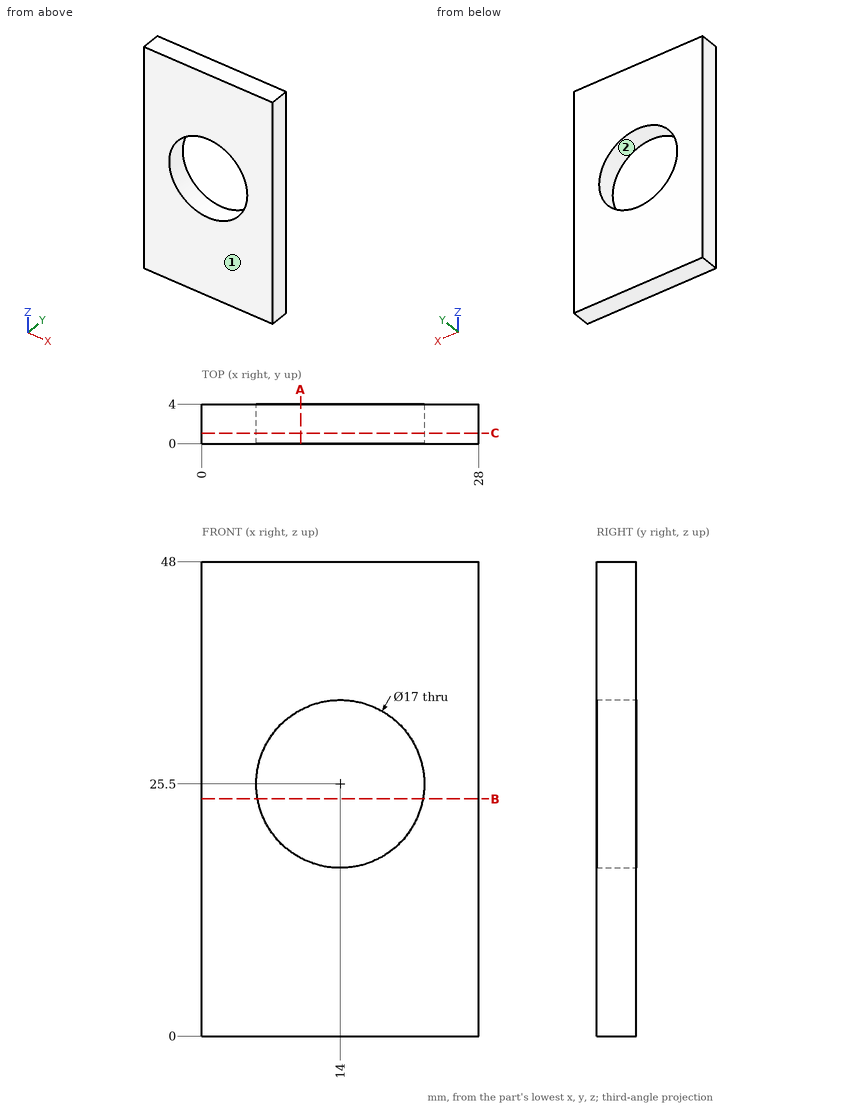
Design review of the part shown in the three views and the two pictorial views. Dimensions are in mm from the part's minimum x, y and z. Round coordinates to 2 decimals unless told otherwise and drop trailing zeros. Order: outer loops, then holes, each group sorted by start corner. A loop starts at its lowest first (then second) coordinate and runs counter-clockwise, first axis right, second up.
(1) Take a section at B-B, the plane z = 24. State the section outline as (x, y) points, plus the area to 3 significant figures.
Working result:
outline: (0, 0) - (5.63, 0) - (5.63, 4) - (0, 4) - close; (22.37, 0) - (28, 0) - (28, 4) - (22.37, 4) - close
area: 45.1 mm2
(2) For P1, Ø4, axis at x = 6.5, z = 10, coming from the -Y side; P2, Ø15.5, axis at x = 14, z = 25.5, coming from the -Y side, all flat-tipped, find the tip position at first contact; note any pin that passes through.
Working result:
P1: stops at y = 0
P2: passes through
(3) Take a section at C-C, the plane y = 1.05. State the section outline as (x, z) points, plus the area to 3 significant figures.
Working result:
outline: (0, 0) - (28, 0) - (28, 48) - (0, 48) - close; hole circle Ø17 at (14, 25.5)
area: 1,120 mm2
(4) Mouldability with a two-part tool opening along Z and no side actions: class the marked faces 1 and 2 as released by +Z, released by -Z, zero draft, split by the parting line, or undercut.
Working result:
face 1: zero draft
face 2: undercut
(5) Take a section at A-A, the plane x = 10. State the section outline as (y, z) points.
Working result:
outline: (0, 0) - (4, 0) - (4, 18) - (0, 18) - close; (0, 33) - (4, 33) - (4, 48) - (0, 48) - close
(6) Wall thickness on L1, parallel to Z at x = 14.25, y = 2.2; L2, parallel to X at y = 1.1, z = 25.5; L3, parallel to Z at x = 17.75, y = 0.45: over which ranges is each line inside the solid? List them lowest first.
Working result:
L1: z = 0 to 17, 34 to 48
L2: x = 0 to 5.5, 22.5 to 28
L3: z = 0 to 17.87, 33.13 to 48
